from build123d import *

# Parameters (mm, degrees)
SKETCH1_W           = 146
SKETCH1_H           = 105
BOSS_EXTRUDE1_DEPTH = 3
SKETCH2_R           = 1.7
SKETCH2_W           = 3
SKETCH2_H           = 15
CUT_EXTRUDE1_DEPTH  = 3


with BuildPart() as part:
    # Sketch1 → Boss-Extrude1 (new body)
    with BuildSketch(Plane(origin=(0, 0, 0), x_dir=(1, 0, 0), z_dir=(0, 1, 0))):
        Rectangle(SKETCH1_W, SKETCH1_H)
    extrude(amount=BOSS_EXTRUDE1_DEPTH)

    # Sketch2 → Cut-Extrude1 (cut)
    with BuildSketch(Plane(origin=(0, 3, 0), x_dir=(1, 0, 0), z_dir=(0, 1, 0))):
        with Locations(Location((-46.5, 45.5, 0), (0, 0, 270))):
            Circle(SKETCH2_R)
        with Locations(Location((46.5, 45.5, 0), (0, 0, 270))):
            Circle(SKETCH2_R)
        with Locations(Location((46.5, -9.5, 0), (0, 0, 270))):
            Circle(SKETCH2_R)
        with Locations(Location((-46.5, -9.5, 0), (0, 0, 270))):
            Circle(SKETCH2_R)
        with Locations(Location((-30.75, -16.278395091, 0), (0, 0, 270))):
            Circle(SKETCH2_R)
        with Locations(Location((30.75, -16.278395091, 0), (0, 0, 270))):
            Circle(SKETCH2_R)
        with Locations(Location((30.75, -42.478395091, 0), (0, 0, 270))):
            Circle(SKETCH2_R)
        with Locations(Location((-30.75, -42.478395091, 0), (0, 0, 270))):
            Circle(SKETCH2_R)
        with Locations((-71.5, -30)):
            Rectangle(SKETCH2_W, SKETCH2_H)
        with Locations((-71.5, 11.27)):
            Rectangle(SKETCH2_W, SKETCH2_H)
        with Locations((71.5, 11.27)):
            Rectangle(SKETCH2_W, SKETCH2_H)
        with Locations((71.5, -30)):
            Rectangle(SKETCH2_W, SKETCH2_H)
    extrude(amount=-CUT_EXTRUDE1_DEPTH, mode=Mode.SUBTRACT)


solid = part.part
Could you check a few things on this model? Use its own coordinates, in mm. A direction names the side the tool comes from. Give positions to 0.01 mm unless a question says otherwise; leave off trailing zeros. Order: outer loops, then holes, each group sorted by start corner. A loop starts at its lowest first (then second) coordinate and runs counter-clockwise, first axis right, second up.
1. Suppose I cut it at B-B (y = 2.55). Give the number of separate pieces and of enclosed holes in the cut face, plus the area to 3 significant figures.
2. Suppose I cut it at C-C (z = -45.5). List the corners of the cut face in (x, y) for me.
3. Suppose I cut it at A-A (x = 46.5). List the corners of the cut face in (y, z) for me.
4. For faces 5 (the flat face through (70, 2, -11)), 6 (the flat face through (-70, 2, 30)), 7 (the cylindrical face through (44.84, 1.52, 9.13)), which set-ups out of +Z, -Z, +X, -X, +Y, -Y let a thin tool reach every point of the face, with its end or its side?
5. Suppose I cut it at D-D (z = 28). List the corners of the cut face in (x, y) for me, plus the area to 3 significant figures.
6. We'd pull the mould along Z, two halves only. Please class faces 1 (the flat face through (-1, 1, 52.5)), 2 (the flat face through (-72, 2, 37.5)), 3 (the flat face through (-73, 1, 45)), 4 (the cylindrical face through (-31.784, 1.521, 41.129)): pulls with the +Z half, pulls with the -Z half, needs draft (parallel to the pull), parting line crosses it, or undercut.
7. I need wall thicknesses on L1, parallel to X at y = 0.95, z = -45.5; L2, parallel to X at y = 0.3, z = 31. Which ranges of each line are inside material? Lowest first, please.
8. Will these pins go through, and if not, where does the flat tip stop? P1, Ø2, axis at x = 30.75, z = 42.48, coming from the -Y side; P2, Ø0.9, axis at y = 2, z = 33.5, coming from the -X side.
Solved:
1. separate pieces: 1
1. enclosed holes: 8
1. area: 15,100 mm2
2. outline: (-73, 0) - (-48.2, 0) - (-48.2, 3) - (-73, 3) - close; (-44.8, 0) - (44.8, 0) - (44.8, 3) - (-44.8, 3) - close; (48.2, 0) - (73, 0) - (73, 3) - (48.2, 3) - close
3. outline: (0, -52.5) - (3, -52.5) - (3, -47.2) - (0, -47.2) - close; (0, -43.8) - (3, -43.8) - (3, 7.8) - (0, 7.8) - close; (0, 11.2) - (3, 11.2) - (3, 52.5) - (0, 52.5) - close
4. face 5: +X, +Y, -Y
4. face 6: -X, +Y, -Y
4. face 7: +Y, -Y
5. outline: (-70, 0) - (70, 0) - (70, 3) - (-70, 3) - close
5. area: 420 mm2
6. face 1: pulls with the +Z half
6. face 2: undercut
6. face 3: needs draft
6. face 4: undercut
7. L1: x = -73 to -48.2, -44.8 to 44.8, 48.2 to 73
7. L2: x = -70 to 70
8. P1: passes through
8. P2: stops at x = -70
